```python
from build123d import *

# Parameters (mm, degrees)
SKETCH1_R           = 6
SKETCH1_R_2         = 2
BOSS_EXTRUDE1_DEPTH = 3
SKETCH2_W           = 3
SKETCH2_H           = 57
BOSS_EXTRUDE2_DEPTH = 12
CUT_EXTRUDE1_REACH  = 64.137
SKETCH3_R           = 2
FILLET1_R           = 3
FILLET2_R           = 3.9
FILLET3_R           = 2


with BuildPart() as part:
    # Sketch1 → Boss-Extrude1 (new body)
    # profile 1 of 2: a face of its own
    with BuildSketch(Plane(origin=(0, 0, 0), x_dir=(1, 0, 0), z_dir=(0, 1, 0))):
        with BuildLine():
            Line((-6, 16), (-6, 0))
            ThreePointArc((-6, 0), (0, 6), (6, 0))
            Line((6, 0), (6, 16))
            Line((6, 16), (-6, 16))
        make_face()
    # profile 2 of 2: a face of its own
    with BuildSketch(Plane(origin=(0, 0, 0), x_dir=(1, 0, 0), z_dir=(0, 1, 0))):
        Circle(SKETCH1_R)
        with Locations(Location((0, 0, 0), (0, 0, 270))):
            Circle(SKETCH1_R_2, mode=Mode.SUBTRACT)
    extrude(amount=BOSS_EXTRUDE1_DEPTH)

    # Sketch2 → Boss-Extrude2 (add)
    with BuildSketch(Plane(origin=(6, 0, 0), x_dir=(0, 0, -1), z_dir=(1, 0, 0))):
        with Locations((10.5, 31.5)):
            Rectangle(SKETCH2_W, SKETCH2_H)
    extrude(amount=-BOSS_EXTRUDE2_DEPTH)

    # Sketch3 → Cut-Extrude1 (cut, up to next)
    with BuildSketch(Plane.XY.offset(-9), mode=Mode.PRIVATE) as cut_extrude1_sk1:
        with BuildLine():
            Line((-6, 60), (-6, 54))
            ThreePointArc((-6, 54), (-4.242640687, 58.242640687), (0, 60))
            Line((0, 60), (-6, 60))
        make_face()
    cut_extrude1_tool1 = extrude(cut_extrude1_sk1.sketch, amount=-CUT_EXTRUDE1_REACH, mode=Mode.PRIVATE) & part.part
    # Sketch3 → Cut-Extrude1 (cut, up to next)
    with BuildSketch(Plane.XY.offset(-9), mode=Mode.PRIVATE) as cut_extrude1_sk2:
        with BuildLine():
            ThreePointArc((0, 60), (4.242640687, 58.242640687), (6, 54))
            Line((6, 54), (6, 60))
            Line((6, 60), (0, 60))
        make_face()
    cut_extrude1_tool2 = extrude(cut_extrude1_sk2.sketch, amount=-CUT_EXTRUDE1_REACH, mode=Mode.PRIVATE) & part.part
    # Sketch3 → Cut-Extrude1 (cut, up to next)
    with BuildSketch(Plane.XY.offset(-9), mode=Mode.PRIVATE) as cut_extrude1_sk3:
        with Locations((0, 54)):
            Circle(SKETCH3_R)
    cut_extrude1_tool3 = extrude(cut_extrude1_sk3.sketch, amount=-CUT_EXTRUDE1_REACH, mode=Mode.PRIVATE) & part.part
    add(cut_extrude1_tool1.solids().sort_by_distance((-4.659792, 58.659792, -9))[0], mode=Mode.SUBTRACT)
    add(cut_extrude1_tool2.solids().sort_by_distance((4.659792, 58.659792, -9))[0], mode=Mode.SUBTRACT)
    add(cut_extrude1_tool3.solids().sort_by_distance((0, 54, -9))[0], mode=Mode.SUBTRACT)

    # Fillet1
    fillet1_edges = [part.edges().sort_by_distance(p)[0] for p in [
        (0, 3, -9),
    ]]
    fillet(fillet1_edges, radius=FILLET1_R)

    # Fillet2
    fillet2_edges = [part.edges().sort_by_distance(p)[0] for p in [
        (0, 3, -12),
    ]]
    fillet(fillet2_edges, radius=FILLET2_R)

    # Fillet3
    fillet3_edges = [part.edges().sort_by_distance(p)[0] for p in [
        (0, 3, -16),
    ]]
    fillet(fillet3_edges, radius=FILLET3_R)


solid = part.part
```
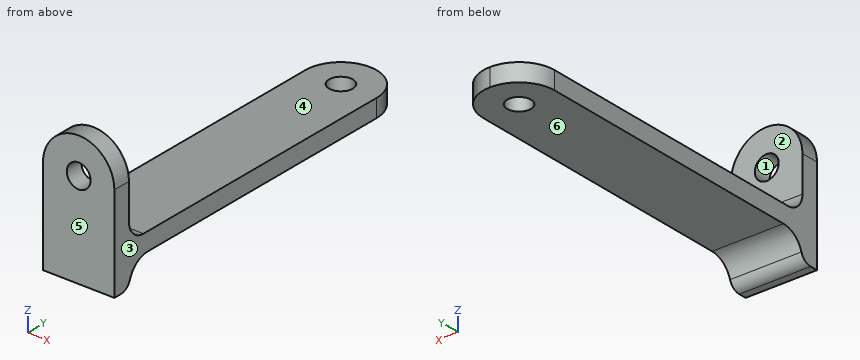
CAD build for the part. Positions are in the model's coordinates, mm. Face numbers are marked on the shaded views. A direction names the side the tool comes from. Round coordinates to 2 decimals unless told otherwise and drop trailing zeros. Order: outer loops, then holes, each group sorted by start corner. A loop starts at its lowest first (then second) coordinate and runs counter-clockwise, first axis right, second up. Notation, with made-up numbers: (45.5, 20) -> (92.5, 20) arc R23 cw to (92.5, 44) -> close; hole circle Ø6 at (18.25, -25.75). An arc over 180 degrees is marked (long way). Write item = value, one per line.
(1) Cut at A-A (y = 37.5). Write the cut outline in (x, z).
Answers follow:
outline = (-6, -12) -> (6, -12) -> (6, -9) -> (-6, -9) -> close
(2) Cut at B-B (z = -13.25). Write the cut outline in (x, y), plus the area to 3 significant figures.
Answers follow:
outline = (-6, 0) -> (6, 0) -> (6, 4.04) -> (-6, 4.04) -> close
area = 48.5 mm²
(3) Drill centre lines: L1, parallel to Y at x = 4.5, z = 0; L2, parallel to Z at x = 2.5, y = 55; L3, parallel to Y at x = 5, z = -14.25. Where is each one in solid material? Low to high.
Answers follow:
L1 = 0 to 3
L2 = -12 to -9
L3 = 0 to 3.37
(4) Flat gauge pins, fed straight in: P1, Ø2.5, axis at x = 0, y = 54, coming from the -Z side (3 decimals); P2, Ø1.5, axis at x = -2.5, y = 19.5, coming from the +Z side; P3, Ø2, axis at x = -3, z = -5, coming from the +Y side; P4, Ø1, axis at x = -4, z = -11.5, coming from the +Y side. Where does each tip first touch, or does it go through?
Answers follow:
P1 = through
P2 = -9
P3 = 3
P4 = 58.87
(5) 3-axis set-ups, long thin cutter, end or side, ignore diameter. For the marked faces 4, 5 and 6: which of +Z, -Z, +X, -X, +Y, -Y reach the whole face in a straight line?
Answers follow:
face_4 = +Z, +X, -X, +Y
face_5 = +Z, -Z, +X, -X, -Y
face_6 = -Z, +X, -X, +Y
(6) Pull direction X, two halves, no side cores. Call the marked faces 1, 2 and 3: +X half, -X half, draft (parallel to the pull), parting line (faces both ways), or undercut.
Answers follow:
face_1 = undercut
face_2 = draft
face_3 = +X half
